Could you check a few things on this model? Use its own coordinates, in mm. A direction names the side the tool comes from. Round coordinates to 2 decimals unless told otherwise and drop trailing zeros. Write each loop counter-clockwise with the first axis right and the second up, starting at its lowest first coordinate (ties: lowest second). Pieces come first, ordered by that corner, then holes. Notation, with made-up numbers: (46, 83) - (67, 83) arc R17 cw to (67, 115) - close; hole circle Ø1 at (-11, 46.5). An arc over 180 degrees is marked (long way). Write each question's results on one line, items separated by ' | '. Start each with the question number.
(1) On a 3-axis mill with a long thin cutter (end or side, diameter ignored), from which of +Z, -Z, +X, -X, +Y, -Y can I reach the whole of each face in a straight line? I mean faces 1 (the flat face through (0, -355, -27)), 2 (the flat face through (0, -355, -30)). Say none if no direction works.
(2) For P1, Ø12, axis at x = -12, z = 12, coming from the -Y side, with a flat end and sliding along its axis, tell me the tip position at first contact or that it passes through.
(3) Imagine slicing it at A-A on z = -18. Write out the boundary of the cut face in (x, y).
(4) Thinking about a two-plate mould opening in X: for faces 3 (the flat face through (-20, -355, 0)), 4 (the flat face through (18, 0, 0)), 5 (the flat face through (-17, -355, 0)), which applies, +X half, -X half, draft (parallel to the pull), parting line (faces both ways), or undercut?
(5) Imagine slicing it at C-C on y = -570. Write out the boundary of the cut face in (x, z).
(6) Imagine slicing it at B-B on x = 8. Write out the boundary of the cut face in (y, z), then the cut area to 3 significant figures.
(7) Please list where these lines run through material, in increasing order: line 1 (Z direction, x = -9.5, y = -361.5); line 2 (X direction, y = -259.5, z = 0); line 3 (X direction, y = -668, z = -25). Write a range as [from, to].
```python
from build123d import *

# Parameters (mm, degrees)
F1_DEPTH = 720


with BuildPart() as f1:
    # F0 (on Front) → F1 (new body)
    with BuildSketch(Plane.XZ):
        with BuildLine():
            Line((14, 30), (-14, 30))
            ThreePointArc((-14, 30), (-18.242641, 28.242641), (-20, 24))
            Line((-20, 24), (-20, -24))
            ThreePointArc((-20, -24), (-18.242641, -28.242641), (-14, -30))
            Line((-14, -30), (14, -30))
            ThreePointArc((14, -30), (18.242641, -28.242641), (20, -24))
            Line((20, -24), (20, 24))
            ThreePointArc((20, 24), (18.242641, 28.242641), (14, 30))
        make_face()
        with BuildLine():
            Line((-17, -24), (-17, 24))
            ThreePointArc((-17, 24), (-16.12132, 26.12132), (-14, 27))
            Line((-14, 27), (14, 27))
            ThreePointArc((14, 27), (16.12132, 26.12132), (17, 24))
            Line((17, 24), (17, -24))
            ThreePointArc((17, -24), (16.12132, -26.12132), (14, -27))
            Line((14, -27), (-14, -27))
            ThreePointArc((-14, -27), (-16.12132, -26.12132), (-17, -24))
        make_face(mode=Mode.SUBTRACT)
    extrude(amount=F1_DEPTH)


solid = f1.part
```
Response:
1) face 1: +Y, -Y | face 2: -Z, +X, -X, +Y, -Y
2) P1: y = -720
3) outline: (-20, -720) - (-17, -720) - (-17, 0) - (-20, 0) - close; (17, -720) - (20, -720) - (20, 0) - (17, 0) - close
4) face 3: -X half | face 4: draft | face 5: undercut
5) outline: (-20, -24) arc R6 ccw to (-14, -30) - (14, -30) arc R6 ccw to (20, -24) - (20, 24) arc R6 ccw to (14, 30) - (-14, 30) arc R6 ccw to (-20, 24) - close; hole (-17, -24) arc R3 ccw to (-14, -27) - (14, -27) arc R3 ccw to (17, -24) - (17, 24) arc R3 ccw to (14, 27) - (-14, 27) arc R3 ccw to (-17, 24) - close
6) outline: (-720, -30) - (0, -30) - (0, -27) - (-720, -27) - close; (-720, 27) - (0, 27) - (0, 30) - (-720, 30) - close | area: 4,320 mm²
7) line 1: [-30, -27], [27, 30] | line 2: [-20, -17], [17, 20] | line 3: [-19.92, -16.83], [16.83, 19.92]
